Could you check a few things on this model? Use its own coordinates, in mm. Round coordinates to 2 decimals unless told otherwise and drop trailing zeros. Loops run counter-clockwise (first coordinate to the right, second up) from the corner with the lowest first, then second, coordinate; pieces in that order, holes last. Notation, with made-up numbers: M 0,2 L 22,2 A17 cw 22,8 Z; hole C 59,38 d9. An arc over 180 degrees is marked long. Answer in a Markdown table with one row per item.
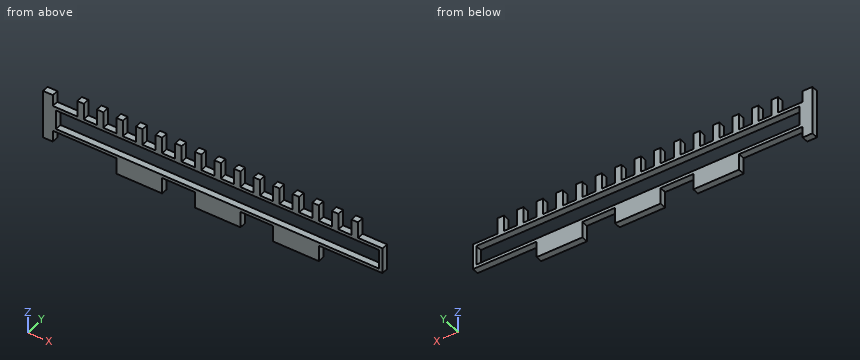
```python
from build123d import *

# Parameters (mm, degrees)
SKETCH1_W           = 101
SKETCH1_H           = 8
SKETCH1_W_2         = 99
SKETCH1_H_2         = 6
BOSS_EXTRUDE1_DEPTH = 2
SKETCH2_W           = 3
SKETCH2_H           = 15
SKETCH2_W_2         = 2
SKETCH2_H_2         = 5
SKETCH2_W_3         = 14
BOSS_EXTRUDE2_DEPTH = 2


with BuildPart() as part:
    # Sketch1 → Boss-Extrude1 (new body)
    with BuildSketch(Plane(origin=(0, 0, 0), x_dir=(1, 0, 0), z_dir=(0, 1, 0))):
        Rectangle(SKETCH1_W, SKETCH1_H)
        Rectangle(SKETCH1_W_2, SKETCH1_H_2, mode=Mode.SUBTRACT)
    extrude(amount=BOSS_EXTRUDE1_DEPTH)

    # Sketch2 → Boss-Extrude2 (add)
    with BuildSketch(Plane(origin=(0, 0, 0), x_dir=(1, 0, 0), z_dir=(0, 1, 0))):
        with Locations((-52, 0)):
            Rectangle(SKETCH2_W, SKETCH2_H)
        with Locations((-42, -6.5)):
            Rectangle(SKETCH2_W_2, SKETCH2_H_2)
        with Locations((-36, -6.5)):
            Rectangle(SKETCH2_W_2, SKETCH2_H_2)
        with Locations((-30, -6.5)):
            Rectangle(SKETCH2_W_2, SKETCH2_H_2)
        with Locations((-24, -6.5)):
            Rectangle(SKETCH2_W_2, SKETCH2_H_2)
        with Locations((-18, -6.5)):
            Rectangle(SKETCH2_W_2, SKETCH2_H_2)
        with Locations((-12, -6.5)):
            Rectangle(SKETCH2_W_2, SKETCH2_H_2)
        with Locations((-6, -6.5)):
            Rectangle(SKETCH2_W_2, SKETCH2_H_2)
        with Locations((0, -6.5)):
            Rectangle(SKETCH2_W_2, SKETCH2_H_2)
        with Locations((6, -6.5)):
            Rectangle(SKETCH2_W_2, SKETCH2_H_2)
        with Locations((12, -6.5)):
            Rectangle(SKETCH2_W_2, SKETCH2_H_2)
        with Locations((18, -6.5)):
            Rectangle(SKETCH2_W_2, SKETCH2_H_2)
        with Locations((24, -6.5)):
            Rectangle(SKETCH2_W_2, SKETCH2_H_2)
        with Locations((30, -6.5)):
            Rectangle(SKETCH2_W_2, SKETCH2_H_2)
        with Locations((36, -6.5)):
            Rectangle(SKETCH2_W_2, SKETCH2_H_2)
        with Locations((42, -6.5)):
            Rectangle(SKETCH2_W_2, SKETCH2_H_2)
        with Locations((-24, 6.5)):
            Rectangle(SKETCH2_W_3, SKETCH2_H_2)
        with Locations((0, 6.5)):
            Rectangle(SKETCH2_W_3, SKETCH2_H_2)
        with Locations((24, 6.5)):
            Rectangle(SKETCH2_W_3, SKETCH2_H_2)
    extrude(amount=BOSS_EXTRUDE2_DEPTH)


solid = part.part
```
1) Will these pins go through, and if not, where does the flat tip stop? P1, Ø1, axis at y = 0.5, z = 7.5, coming from the +X side; P2, Ø6, axis at x = 17.5, z = 0.5, coming from the +Y side; P3, Ø0.6, axis at x = 32, y = 1, coming from the +Z side.
Computed:
| item | result |
|---|---|
| P1 | stops at x = 43 |
| P2 | stops at y = 2 |
| P3 | stops at z = 4 |
2) I want a section at C-C, the plane z = 5. State how many separate pieces and enclosed holes the cut face has, plus the area to 3 significant figures.
Computed:
| item | result |
|---|---|
| separate pieces | 16 |
| enclosed holes | 0 |
| area | 66.0 mm² |
3) I want a section at A-A, the plane x = -39. Please give me the cut outline in (y, z), plus the area to 3 significant figures.
Computed:
| item | result |
|---|---|
| outline | M 0,-4 L 2,-4 L 2,-3 L 0,-3 Z; M 0,3 L 2,3 L 2,4 L 0,4 Z |
| area | 4.00 mm² |
4) I need wall thicknesses on line 1 (X direction, y = 1.8, z = -6); line 2 (Z direction, x = 36.5, y = 0.8); line 3 (Z direction, x = 2.5, y = 1.8). Which ranges of each line are inside material? Lowest first, please.
Computed:
| item | result |
|---|---|
| line 1 | x = -53.5 to -50.5, -31 to -17, -7 to 7, 17 to 31 |
| line 2 | z = -4 to -3, 3 to 9 |
| line 3 | z = -9 to -3, 3 to 4 |
5) I want a section at B-B, the plane z = 0.5. Please give me the cut outline in (x, y), plus the area to 3 significant figures.
Computed:
| item | result |
|---|---|
| outline | M -53.5,0 L -49.5,0 L -49.5,2 L -53.5,2 Z; M 49.5,0 L 50.5,0 L 50.5,2 L 49.5,2 Z |
| area | 10.0 mm² |
